The listing builds one solid part. Answer for the finished solid, in the listing's coordinates (mm). Give positions to 0.01 mm unless a question says otherwise; leave off trailing zeros. Write each loop counter-clockwise with the first axis right and the second up, starting at its lowest first coordinate (ties: lowest second). Pieces come first, ordered by that corner, then holes. Notation, with made-up numbers: (66.25, -24) - (72.25, -24) arc R27 ccw to (72.25, 1) - close; hole circle Ø1 at (78, 66). An arc over 180 degrees is marked (long way). Answer in a Markdown table with one row per item. Add a question column.
from build123d import *

# Parameters (mm, degrees)
SKETCH1_W           = 20
SKETCH1_H           = 40
BOSS_EXTRUDE1_DEPTH = 105.33
CUT_EXTRUDE1_DEPTH  = 106.33


with BuildPart() as part:
    # Sketch1 → Boss-Extrude1 (new body)
    with BuildSketch(Plane.XY):
        with Locations((10, 20)):
            Rectangle(SKETCH1_W, SKETCH1_H)
    extrude(amount=BOSS_EXTRUDE1_DEPTH)

    # Sketch2 → Cut-Extrude1 (cut, through all)
    with BuildSketch(Plane.XY.offset(105.33)):
        Polygon((5.12, 40), (6.94, 38.18), (4.5, 38.18), (4.5, 36.475807358), (7.165807358, 33.81), (12.834192642, 33.81), (15.5, 36.475807358), (15.5, 38.18), (13.06, 38.18), (14.88, 40), align=None)
        Polygon((18.18, 35.5), (18.18, 33.06), (20, 34.88), (20, 25.12), (18.18, 26.94), (18.18, 24.5), (16.475807358, 24.5), (13.81, 27.165807358), (13.81, 32.834192642), (16.475807358, 35.5), align=None)
        Polygon((20, 14.88), (18.18, 13.06), (18.18, 15.5), (16.475807358, 15.5), (13.81, 12.834192642), (13.81, 7.165807358), (16.475807358, 4.5), (18.18, 4.5), (18.18, 6.94), (20, 5.12), align=None)
        Polygon((15.5, 1.82), (13.06, 1.82), (14.88, 0), (5.12, 0), (6.94, 1.82), (4.5, 1.82), (4.5, 3.524192642), (7.165807358, 6.19), (12.834192642, 6.19), (15.5, 3.524192642), align=None)
        Polygon((1.82, 4.5), (1.82, 6.94), (0, 5.12), (0, 14.88), (1.82, 13.06), (1.82, 15.5), (3.524192642, 15.5), (6.19, 12.834192642), (6.19, 7.165807358), (3.524192642, 4.5), align=None)
        Polygon((0, 25.12), (1.82, 26.94), (1.82, 24.5), (3.524192642, 24.5), (6.19, 27.165807358), (6.19, 32.834192642), (3.524192642, 35.5), (1.82, 35.5), (1.82, 33.06), (0, 34.88), align=None)
    extrude(amount=-CUT_EXTRUDE1_DEPTH, mode=Mode.SUBTRACT)


solid = part.part
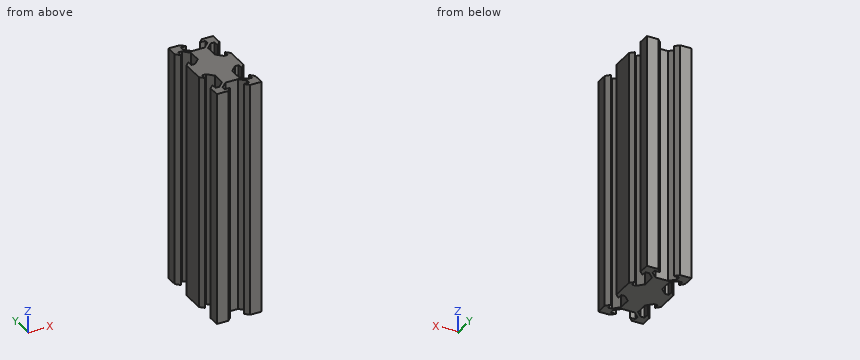
1. Straight lines are drawn through the part: L1, parallel to Y at x = 2.25, z = 41.5; L2, parallel to X at y = 3.5, z = 71.5; L3, parallel to X at y = 35, z = 96. For each, find the intervals that lie inside material, in ascending order. Write a range as [from, to].
2. Section B-B (y = 9.5) is taken. Give the vertices of the cut face in (x, z).
3. Given pin 1 Ø3 at (x, z) = (12, 79.5) entering from -Y; pin 2 Ø1.7 at (y, z) = (30.5, 63.5) entering from -X; pin 3 Ø4.5 at (x, z) = (10, 65) entering from -Y, each flat-ended and moving along its own axis, determine where each tip first touches the part or whether it passes through.
4. Section A-A (x = 9.75) is taken. Give the vertices of the cut face in (y, z), and give its area (3 significant figures).
Geometry check:
| question | item | result |
|---|---|---|
| 1 | L1 | [0, 4.5], [15.5, 24.5], [35.5, 40] |
| 1 | L2 | [0, 4.5], [15.5, 20] |
| 1 | L3 | [0, 1.82], [4.02, 5.98], [14.02, 15.98], [18.18, 20] |
| 2 | outline | (6.19, 0) - (13.81, 0) - (13.81, 105.33) - (6.19, 105.33) - close |
| 3 | pin 1 | y = 1.38 |
| 3 | pin 2 | x = 6.19 |
| 3 | pin 3 | y = 6.19 |
| 4 | outline | (6.19, 0) - (33.81, 0) - (33.81, 105.33) - (6.19, 105.33) - close |
| 4 | area | 2,910 mm² |
